```python
from build123d import *

# Parameters (mm, degrees)
F1_DEPTH = 5
F2_W     = 20
F2_H     = 5
F2_W_2   = 6.8679952621
F2_H_2   = 70
F3_DEPTH = 25
F4_R     = 1
F6_DEPTH = 30.001


with BuildPart() as f1:
    # F0 (on Front) → F1 (new body)
    with BuildSketch(Plane.XZ):
        Polygon((10, 15), (0, 15), (-10, 15), (-10, 10), (-16.8679952621, -10), (-16.8679952621, -80), (0, -80), (10, -80), (80, -10), (10, 10), align=None)
    extrude(amount=-F1_DEPTH)

    # F2 (on face) → F3 (join)
    with BuildSketch(Plane.XZ):
        with Locations((0, 12.5)):
            Rectangle(F2_W, F2_H)
        Polygon((10, -80), (80, -10), (10, -10), align=None)
        with Locations((-13.4339976311, -45)):
            Rectangle(F2_W_2, F2_H_2)
    extrude(amount=F3_DEPTH)

    # F4
    f4_edges = [f1.edges().sort_by_distance(p)[0] for p in [
        (0, 0, 10),
        (-13.433998, 0, -10),
        (45, 0, -10),
        (10, 0, -45),
        (-10, 0, -45),
        (0, -25, 10),
        (45, -25, -10),
        (10, -25, -45),
        (-13.433998, -25, -10),
        (-10, -25, -45),
    ]]
    fillet(f4_edges, radius=F4_R)

    # F5 (on face) → F6 (cut, through all)
    with BuildSketch(Plane.XZ.offset(25)):
        Polygon((55.8578643763, -20), (20, -20), (20, -55.8578643763), align=None)
    extrude(amount=-F6_DEPTH, mode=Mode.SUBTRACT)


solid = f1.part
```
Input: part model. Units: mm. Frame: model coordinates. A direction names the side the tool comes from. Give positions to 0.01 mm unless a question says otherwise; leave off trailing zeros. Loops run counter-clockwise (first coordinate to the right, second up) from the corner with the lowest first, then second, coordinate; pieces in that order, holes last.
1) Contact query for flat-ended pins moving along their axis: pin 1 (12 mm diameter, centred on x = 22.5, z = -50, fed in from -Y); pin 2 (11.5 mm diameter, centred on x = 33, y = -17.5, fed in from +Z); pin 3 (15 mm diameter, centred on y = -13.5, z = -43, fed in from +X); pin 4 (9 mm diameter, centred on x = 31.5, y = -17.5, fed in from -Z). Output: stop coordinate, or through.
A:
pin 1: stops at y = -25
pin 2: stops at z = -10
pin 3: stops at x = 54.5
pin 4: stops at z = -63
2) Reachability of faces 1 (the flat face through (10, -12, -45)), 2 (the flat face through (38, -10, -20)), 3 (the flat face through (45, -12, -10)), 4 (the flat face through (-10, -10, 12)), 5 (the flat face through (6, 0, -22)) from +Z, -Z, +X, -X, +Y, -Y: full face, straight path, thin tool, end or side. Return the list, or none.
A:
face 1: -Z, -Y
face 2: +Y, -Y
face 3: +Z, +X, -X, -Y
face 4: +Z, -X, +Y, -Y
face 5: -Y
3) Section query B-B on x = -6. Return the cut outline in (y, z).
A:
outline: (-25, 11) arc R1 ccw to (-24, 10) - (-1, 10) arc R1 cw to (0, 9) - (0, -80) - (5, -80) - (5, 15) - (-25, 15) - close
4) Line query: L1, parallel to X at y = -4, z = -42; L2, parallel to Y at x = -6.5, z = -58; L3, parallel to Z at x = 46.5, y = -10.5. Output: solid intervals per line, ascending.
A:
L1: x = -16.87 to -10, 10 to 20, 33.86 to 48
L2: y = 0 to 5
L3: z = -43.5 to -29.36, -20 to -10
5) Mould query, pull axis Z, two halves, no side actions, for faces 6 (the flat face through (20, -10, -38)), 7 (the flat face through (45, 3, 0)), 8 (the flat face through (10, -10, 12)), 9 (the flat face through (37.68, -10.21, -38.18)). Classes: released by +Z, released by -Z, zero draft, split by the parting line, or undercut.
A:
face 6: undercut
face 7: released by +Z
face 8: zero draft
face 9: undercut
6) Section query A-A on y = -22. Return the cut outline in (x, z).
A:
outline: (-16.87, -80) - (-10, -80) - (-10, -10) - (-16.87, -10) - close; (-10, 10) - (10, 10) - (10, 15) - (-10, 15) - close; (10, -80) - (80, -10) - (10, -10) - close; hole (20, -55.86) - (55.86, -20) - (20, -20) - close
7) Section query C-C on x = 24. Return the cut outline in (y, z), and give its area (3 significant figures).
A:
outline: (-25, -66) - (5, -66) - (5, -51.86) - (-25, -51.86) - close; (-25, -20) - (5, -20) - (5, 6) - (0, 6) - (0, -9) arc R1 cw to (-1, -10) - (-24, -10) arc R1 ccw to (-25, -11) - close
area: 804 mm2
8) Section query D-D on z = -71. Return the cut outline in (x, y), and give its area (3 significant figures).
A:
outline: (-16.87, -25) - (-11, -25) arc R1 ccw to (-10, -24) - (-10, -1) arc R1 cw to (-9, 0) - (9, 0) arc R1 cw to (10, -1) - (10, -24) arc R1 ccw to (11, -25) - (19, -25) - (19, 5) - (-16.87, 5) - close
area: 576 mm2
